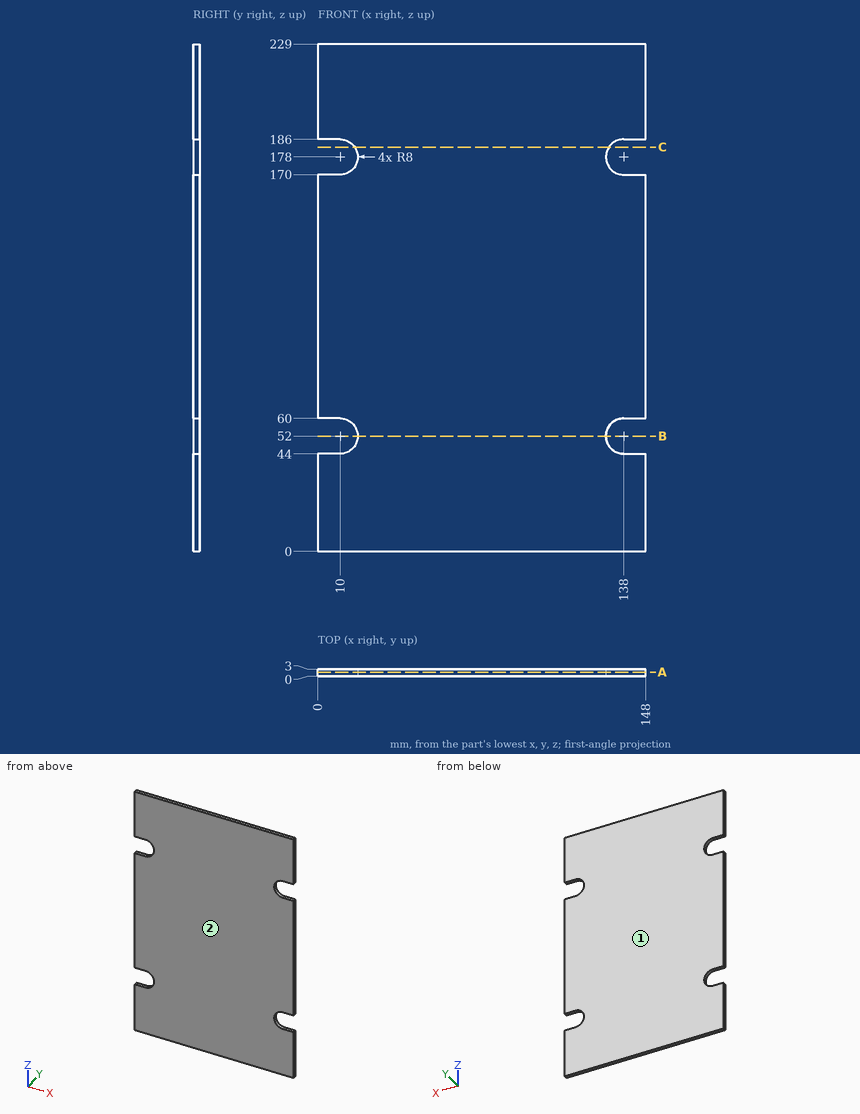
Input: dimensioned drawing with shaded views. Units: mm. Origin: part minimum x, y, z. Round coordinates to 2 decimals unless told otherwise and drop trailing zeros. Loops run counter-clockwise (first coordinate to the right, second up) from the corner with the lowest first, then second, coordinate; pieces in that order, holes last. Notation, with made-up numbers: (25, 6) -> (79, 6) arc R18 ccw to (79, 17) -> close; hole circle Ø4 at (20, -6). An arc over 180 degrees is marked (long way). Answer as a JSON object with one key per item and string values. Group by question number.
1) Draft query along Y for the marked faces 1 and 2. Return one class per face: +Y half, -Y half, draft (parallel to the pull), parting line (faces both ways), or undercut.
2) Section query B-B on z = 52. Output: boundary loops of the cut face in (x, y).
3) Section query A-A on y = 1.8. Output: boundary loops of the cut face in (x, z), plus the area to 3 significant figures.
4) Ray query, L1, parallel to Z at x = 9, y = 2.1; L2, parallel to X at y = 0.55, z = 178; L3, parallel to X at y = 1, z = 57.5. Return the intervals inside material, ascending.
5) Section query C-C on z = 182.5. Output: boundary loops of the cut face in (x, y).
Reply:
{
 "1": {"face 1": "+Y half", "face 2": "-Y half"},
 "2": {"outline": "(18, 0) -> (130, 0) -> (130, 3) -> (18, 3) -> close"},
 "3": {"outline": "(0, 0) -> (148, 0) -> (148, 44) -> (138, 44) arc R8 cw to (138, 60) -> (148, 60) -> (148, 170) -> (138, 170) arc R8 cw to (138, 186) -> (148, 186) -> (148, 229) -> (0, 229) -> (0, 186) -> (10, 186) arc R8 cw to (10, 170) -> (0, 170) -> (0, 60) -> (10, 60) arc R8 cw to (10, 44) -> (0, 44) -> close", "area": "32,800 mm2"},
 "4": {"L1": "z = 0 to 44, 60 to 170, 186 to 229", "L2": "x = 18 to 130", "L3": "x = 15.81 to 132.19"},
 "5": {"outline": "(16.61, 0) -> (131.39, 0) -> (131.39, 3) -> (16.61, 3) -> close"}
}
